from build123d import *

# Parameters (mm, degrees)
SKETCH_1_R               = 7
EXTRUDE_1_DEPTH          = 3
SKETCH_2_W               = 2.1
SKETCH_2_H               = 10
CUT_EXTRUDE_1_DEPTH      = 1.9
SKETCH_3_R               = 1.05
CUT_EXTRUDE_2_DEPTH      = 1
CUT_EXTRUDE_2_DEPTH_BACK = 2.5
SKETCH_4_R               = 0.5
CUT_EXTRUDE_3_DEPTH      = 1
CUT_EXTRUDE_3_DEPTH_BACK = 4
CHAMFER_1_SIZE           = 0.4


with BuildPart() as part:
    # Эскиз1 → Бобышка-Вытянуть1 (new body)
    with BuildSketch(Plane(origin=(0, 0, 0), x_dir=(1, 0, 0), z_dir=(0, 1, 0))):
        Circle(SKETCH_1_R)
    extrude(amount=EXTRUDE_1_DEPTH)

    # Эскиз2 → Вырез-Вытянуть1 (cut)
    with BuildSketch(Plane.XZ):
        Polygon((10.917234456, -5.090702278), (9.867234456, -6.909355626), (1.206980418, -1.909355626), (2.256980418, -0.090702278), align=None)
        with Locations((-7.039e-05, 6.999971048)):
            Rectangle(SKETCH_2_W, SKETCH_2_H)
        Polygon((-9.867375235, -6.909355626), (-10.917375235, -5.090702278), (-2.257121197, -0.090702278), (-1.207121197, -1.909355626), align=None)
    extrude(amount=-CUT_EXTRUDE_1_DEPTH, mode=Mode.SUBTRACT)

    # Эскиз3 → Вырез-Вытянуть2 (cut, two sides)
    with BuildSketch(Plane.XZ) as cut_extrude_2_sk:
        Circle(SKETCH_3_R)
    extrude(amount=CUT_EXTRUDE_2_DEPTH, mode=Mode.SUBTRACT)
    extrude(cut_extrude_2_sk.sketch, amount=-CUT_EXTRUDE_2_DEPTH_BACK, mode=Mode.SUBTRACT)

    # Эскиз4 → Вырез-Вытянуть3 (cut, two sides)
    with BuildSketch(Plane.XZ) as cut_extrude_3_sk:
        with Locations((0, -4)):
            Circle(SKETCH_4_R)
        with Locations((-3.464101615, 2)):
            Circle(SKETCH_4_R)
        with Locations((3.464101615, 2)):
            Circle(SKETCH_4_R)
    extrude(amount=CUT_EXTRUDE_3_DEPTH, mode=Mode.SUBTRACT)
    extrude(cut_extrude_3_sk.sketch, amount=-CUT_EXTRUDE_3_DEPTH_BACK, mode=Mode.SUBTRACT)

    # Фаска1
    chamfer_1_edges = [part.edges().sort_by_distance(p)[0] for p in [
        (-7, 3, 0),
    ]]
    chamfer(chamfer_1_edges, length=CHAMFER_1_SIZE)


solid = part.part
The model under review builds one solid part; all positions refer to its coordinate system, in mm. A direction names the side the tool comes from. Give positions to 0.01 mm unless a question says otherwise; leave off trailing zeros. Loops run counter-clockwise (first coordinate to the right, second up) from the corner with the lowest first, then second, coordinate; pieces in that order, holes last. Notation, with made-up numbers: (87.5, 40.25) -> (130.5, 40.25) arc R31 cw to (130.5, 79.25) -> close; hole circle Ø10 at (-29, -23.5). An arc over 180 degrees is marked (long way). Answer as a JSON object with one key per item and string values. Group by question number.
Q1. Draft analysis for pull direction Z (two halves, no side actions). For faces 4 (the flat face through (-1.74, 0.94, -0.99)), 5 (the flat face through (-1.05, 1, 4)), 6 (the flat face through (0, 1, 2)), state which applies: pulls with the +Z half, pulls with the -Z half, needs draft (parallel to the pull), parting line crosses it, or undercut.
Q2. Take a section at B-B (y = 0.35). Write out the cut boundary in (x, z).
Q3. Take a section at C-C (y = 2.3). Write out the cut boundary in (x, z), plus the area to 3 significant figures.
Q4. Take a section at A-A (x = 0). Write out the cut boundary in (y, z), plus the area to 3 significant figures.
Q5. Wall thickness on line 1 along Z through (x, y) = (0, 1.25); line 2 along Z through (x, y) = (0, 2.45); line 3 along X through (y, z) = (1.05, -0.75): over which ranges is each line inside the solid? List them lowest first.
Q6. Insertion check: pin 1 (1 mm diameter, centred on y = 1.5, z = 5.5, fed in from +X); pin 2 (2 mm diameter, centred on x = 3.5, z = -1, fed in from -Y); pin 3 (1.5 mm diameter, centred on y = 1, z = 3, fed in from -X); pin 4 (1.5 mm diameter, centred on x = 4.5, y = 2, fed in from -Z). Each pin has a flat end and moves straight along its axis. Give the tip position at first contact, or say it passes through.
Q7. Tool access review of faces 1 (the cylindrical face through (-3.83, 1.48, 2.34)), 2 (the flat face through (4, 1.9, -2)), 3 (the flat face through (0, 1.9, 5)): name each direction out of +Z, -Z, +X, -X, +Y, -Y from which nothing blocks a thin tool from reaching the whole face with its end or side.
Answer below:
{
 "1": {"face 4": "undercut", "face 5": "needs draft", "face 6": "pulls with the +Z half"},
 "2": {"outline": "(-6.52, -2.55) -> (-2.26, -0.09) -> (-1.21, -1.91) -> (-5.47, -4.37) arc R7 ccw to (5.47, -4.37) -> (1.21, -1.91) -> (2.26, -0.09) -> (6.52, -2.55) arc R7 ccw to (1.05, 6.92) -> (1.05, 2) -> (-1.05, 2) -> (-1.05, 6.92) arc R7 ccw to start; hole circle Ø1 at (-3.46, 2); hole circle Ø2.1 at (0, 0); hole circle Ø1 at (0, -4); hole circle Ø1 at (3.46, 2)"},
 "3": {"outline": "circle Ø14 at (0, 0); hole circle Ø1 at (-3.46, 2); hole circle Ø2.1 at (0, 0); hole circle Ø1 at (0, -4); hole circle Ø1 at (3.46, 2)", "area": "148 mm2"},
 "4": {"outline": "(0, -7) -> (2.6, -7) -> (3, -6.6) -> (3, -4.5) -> (0, -4.5) -> close; (0, -3.5) -> (3, -3.5) -> (3, 6.6) -> (2.6, 7) -> (1.9, 7) -> (1.9, 2) -> (0, 2) -> (0, 1.05) -> (2.5, 1.05) -> (2.5, -1.05) -> (0, -1.05) -> close", "area": "24.1 mm2"},
 "5": {"line 1": "z = -7 to -4.5, -3.5 to -1.05, 1.05 to 2", "line 2": "z = -7 to -4.5, -3.5 to -1.05, 1.05 to 7", "line 3": "x = -6.96 to -3.4, -1.88 to -0.73, 0.73 to 1.88, 3.4 to 6.96"},
 "6": {"pin 1": "stops at x = 4.9", "pin 2": "stops at y = 0", "pin 3": "stops at x = -6.63", "pin 4": "stops at z = -5.91"},
 "7": {"face 1": "+Y, -Y", "face 2": "-Y", "face 3": "+Z, -Y"}
}
